Part model, mm, in its own coordinate system. Coordinates: 2 decimals unless noted, no trailing zeros. Loops run counter-clockwise (first coordinate to the right, second up) from the corner with the lowest first, then second, coordinate; pieces in that order, holes last. Notation, with made-up numbers: M 9,39.25 L 62,39.25 A21 cw 62,53.25 Z; hole C 38,11.25 d1. An arc over 180 degrees is marked long. Answer as a JSON object with one key per item and string values. Group by question number.
1. Drop flat-ended pins along their axis: pin 1 Ø12 at (x, y) = (74.5, 19) entering from -Z; pin 2 Ø1 at (x, z) = (67.5, 2) entering from -Y (3 decimals). Give the stop position or say it passes through.
2. Drill centre lines: L1, parallel to Y at x = 19.05, z = 1.5 (3 decimals); L2, parallel to X at y = 8.5, z = 2.6 (3 decimals); L3, parallel to Y at x = 20.5, z = 1.25. Where is each one in solid material? Low to high.
3. Saw through at D-D on y = 23. Write the cut outline in (x, z) (3 decimals), then the cut area to 3 significant figures.
4. Saw through at C-C on z = 1.9. Write the cut outline in (x, y) (3 decimals), then the cut area to 3 significant figures.
5. Saw through at A-A on y = 38.1. Write the cut outline in (x, z) (3 decimals), then the cut area to 3 significant figures.
6. Mould opens along Y. For faces 1 (the face through (17.81, 47.544, 1.61)), 2 (the face through (60.325, 16, 2)), 3 (the face through (73, 28.575, 2)) say: released by +Y, released by -Y, zero draft, split by the parting line, or undercut.
7. Saw through at B-B on x = 19.05. Write the cut outline in (y, z) (3 decimals).
Autodesk Inventor part; units mm, degrees
ref_plane "YZ Plane" through (0, 0, 0) normal (1, 0, 0) x (0, 1, 0)
ref_plane "XZ Plane" through (0, 0, 0) normal (0, 1, 0) x (-1, 0, 0)
ref_plane "XY Plane" through (0, 0, 0) normal (0, 0, 1) x (1, 0, 0)
sketch "Sketch1" plane through (0, 0, 0) normal (0, 0, 1) x (1, 0, 0)
  line L0 (0, 0) -> (88.9, 0)
  line L1 (88.9, 0) -> (88.9, 76.2)
  line L2 (88.9, 76.2) -> (0, 76.2)
  line L3 (0, 76.2) -> (0, 0)
  dimension "d9" = 88.9
  dimension "d10" = 76.2
extrude "Extrusion1" add sketch "Sketch1" along normal blind 3.175
sketch "Sketch3" plane through (0, 0, 3.175) normal (0, 0, 1) x (1, 0, 0)
  line L0 (88.9, 0) -> (60.325, 0)
  line L1 (60.325, 0) -> (60.325, 28.575)
  line L2 (60.325, 28.575) -> (88.9, 28.575)
  line L3 (88.9, 28.575) -> (88.9, 0)
  dimension "d12" = 28.575
extrude "Extrusion3" cut sketch "Sketch3" against normal through all
sketch "Sketch4" plane through (0, 0, 3.175) normal (0, 0, 1) x (1, 0, 0)
  line L0 (0, 0) -> (0, 76.2)
  line L1 (60.325, 0) -> (0, 0)
  circle A0 centre (19.05, 38.1) radius 9.525
  dimension "d15" = 19.05
  dimension "d16" = 38.1
  dimension "d17" = 19.05
extrude "Extrusion4" cut sketch "Sketch4" against normal through all
fillet "Fillet1" radius 3.175 5 edges at (0, 76.2, 1.5875) (0, 0, 1.5875) (60.325, 0, 1.5875) (88.9, 28.575, 1.5875) (88.9, 76.2, 1.5875)
properties part number "Plate_VerticalRollerMount_Top" material "Aluminum-6061"
Outcome:
{
 "1": {"pin 1": "passes through", "pin 2": "stops at y = 28.575"},
 "2": {"L1": "y = 0 to 28.575, 47.625 to 76.2", "L2": "x = 0 to 60.325", "L3": "y = 0 to 28.69, 47.51 to 76.2"},
 "3": {"outline": "M 0,0 L 60.325,0 L 60.325,3.175 L 0,3.175 Z", "area": "192 mm²"},
 "4": {"outline": "M 0,3.175 A3.175 ccw 3.175,0 L 57.15,0 A3.175 ccw 60.325,3.175 L 60.325,28.575 L 85.725,28.575 A3.175 ccw 88.9,31.75 L 88.9,73.025 A3.175 ccw 85.725,76.2 L 3.175,76.2 A3.175 ccw 0,73.025 Z; hole C 19.05,38.1 d19.05", "area": "5,660 mm²"},
 "5": {"outline": "M 0,0 L 9.525,0 L 9.525,3.175 L 0,3.175 Z; M 28.575,0 L 88.9,0 L 88.9,3.175 L 28.575,3.175 Z", "area": "222 mm²"},
 "6": {"face 1": "undercut", "face 2": "zero draft", "face 3": "released by -Y"},
 "7": {"outline": "M 0,0 L 28.575,0 L 28.575,3.175 L 0,3.175 Z; M 47.625,0 L 76.2,0 L 76.2,3.175 L 47.625,3.175 Z"}
}
